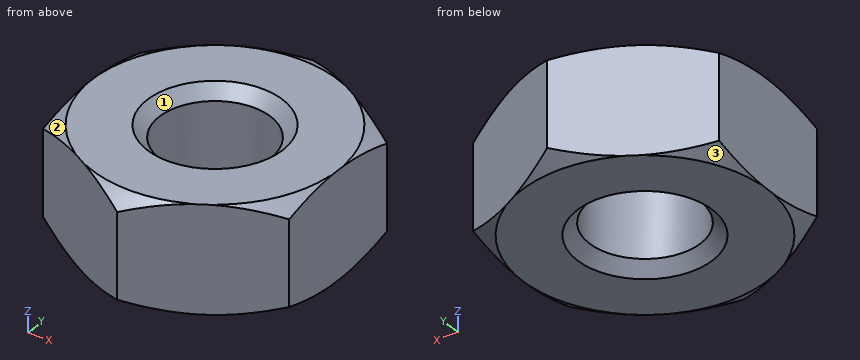
from build123d import *

# Parameters (mm, degrees)
SKETCH2_R           = 1.25
BOSS_EXTRUDE1_DEPTH = 1.2
CHAMFER1_SIZE       = 0.2705


with BuildPart() as part:
    # Sketch2 → Boss-Extrude1 (new body, symmetric)
    with BuildSketch(Plane.XY):
        Polygon((2.75, 1.58771324), (2.75, -1.58771324), (0, -3.175426481), (-2.75, -1.58771324), (-2.75, 1.58771324), (0, 3.175426481), align=None)
        Circle(SKETCH2_R, mode=Mode.SUBTRACT)
    extrude(amount=BOSS_EXTRUDE1_DEPTH, both=True)

    # Sketch4 → Cut-Revolve2 (revolve, cut)
    with BuildSketch(Plane(origin=(0, 0, 0), x_dir=(0, 0, -1), z_dir=(1, 0, 0))):
        Polygon((1.2, 2.75), (1.2, 4.328660734), (0.2885598, 4.328660734), align=None)
    cut_revolve2 = revolve(axis=Axis((0, 0, 2.99453507), (0, 0, -1)), mode=Mode.SUBTRACT)

    # Mirror1: Cut-Revolve2 across plane
    add(cut_revolve2.mirror(Plane.XY), mode=Mode.SUBTRACT)

    # Chamfer1
    chamfer1_edges = [part.edges().sort_by_distance(p)[0] for p in [
        (-1.25, 0, -1.2),
        (-1.25, 0, 1.2),
    ]]
    chamfer(chamfer1_edges, length=CHAMFER1_SIZE)


solid = part.part
Work out the finished part from the listing and answer in its coordinate system (mm). Face numbers are marked on the shaded views. Give positions to 0.01 mm unless a question says otherwise; leave off trailing zeros. Loops run counter-clockwise (first coordinate to the right, second up) from the corner with the lowest first, then second, coordinate; pieces in that order, holes last. Notation, with made-up numbers: M 88,-9.5 L 102,-9.5 A27 ccw 102,13.5 Z; hole C -7.5,79 d8. An arc over 180 degrees is marked long. Use CSV: the item, a comma, the result in double quotes.
1) Consider L1, parallel to Y at x = -0.2, z = 0.05; L2, parallel to Y at x = -1.15, z = 1; L3, parallel to X at y = -0.25, z = 0.45. Determine where each line is inside the solid, lowest interval first.
Answer:
L1,"-3.06 to -1.23, 1.23 to 3.06"
L2,"-2.51 to -0.65, 0.65 to 2.51"
L3,"-2.75 to -1.22, 1.22 to 2.75"
2) Find section A-A on z = -0.4. Write down the section's boundary in (x, y).
Answer:
outline,"M -2.75,-1.59 L 0,-3.18 L 2.75,-1.59 L 2.75,1.59 L 0,3.18 L -2.75,1.59 Z; hole C 0,0 d2.5"
3) Determine the mould class of the marked faces 1, 2 and 3 for opening direction Y: released by +Y, released by -Y, zero draft, split by the parting line, or undercut.
Answer:
face 1,"undercut"
face 2,"released by -Y"
face 3,"released by +Y"
4) Given P1, Ø1.5, axis at x = 0, y = 0, coming from the -Z side, flat-ended and moving along its own axis, determine where the tip first touches the part or whether it passes through.
Answer:
P1,"through"
